Design review of the part built by this model. Coordinates are the model's own, in mm. A direction names the side the tool comes from. Coordinates: 2 decimals unless noted, no trailing zeros. Order: outer loops, then holes, each group sorted by start corner. A loop starts at its lowest first (then second) coordinate and runs counter-clockwise, first axis right, second up. Notation, with made-up numbers: M 83,72 L 127,72 A5 cw 127,78 Z; hole C 15.25,58.5 d4. An arc over 180 degrees is marked long. Answer as a JSON object with one key per item and string values.
from build123d import *

# Parameters (mm, degrees)
MODEL_R             = 19.83955
BOSS_EXTRUDE1_DEPTH = 6.35


with BuildPart() as part:
    # Model → Boss-Extrude1 (new body)
    with BuildSketch(Plane.XY):
        with BuildLine():
            Line((-20.5954, 56.0124), (-20.5954, 81.2129))
            Line((-20.5954, 81.2129), (-14.4452, 81.2129))
            Line((-14.4452, 81.2129), (-14.4452, 107.2136))
            Line((-14.4452, 107.2136), (-20.5954, 107.2136))
            Line((-20.5954, 107.2136), (-20.5954, 132.4124))
            Line((-20.5954, 132.4124), (-14.4452, 132.4124))
            Line((-14.4452, 132.4124), (-14.4452, 151.262))
            Line((-14.4452, 151.262), (-4.2849, 151.262))
            Line((-4.2849, 151.262), (-4.2849, 161.223))
            add(Edge.make_bspline(
                [(2.0647, 167.573), (-1.4529, 167.573), (-4.2849, 164.741), (-4.2849, 161.223)],
                knots=[0.181818182, 0.181818182, 0.181818182, 0.181818182, 0.212121212, 0.212121212, 0.212121212, 0.212121212], degree=3))
            Line((2.0647, 167.573), (27.2651, 167.573))
            add(Edge.make_bspline(
                [(33.6151, 161.223), (33.6151, 164.741), (30.7835, 167.573), (27.2651, 167.573)],
                knots=[0.121212121, 0.121212121, 0.121212121, 0.121212121, 0.151515152, 0.151515152, 0.151515152, 0.151515152], degree=3))
            Line((33.6151, 161.223), (33.6151, 151.262))
            Line((33.6151, 151.262), (43.7754, 151.262))
            Line((43.7754, 151.262), (43.7754, 132.4124))
            Line((43.7754, 132.4124), (49.9256, 132.4124))
            Line((49.9256, 132.4124), (49.9256, 107.2136))
            Line((49.9256, 107.2136), (43.7754, 107.2136))
            Line((43.7754, 107.2136), (43.7754, 81.2129))
            Line((43.7754, 81.2129), (49.9256, 81.2129))
            Line((49.9256, 81.2129), (49.9256, 56.0124))
            Line((49.9256, 56.0124), (43.7754, 56.0124))
            Line((43.7754, 56.0124), (43.7754, 37.1628))
            Line((43.7754, 37.1628), (33.6151, 37.1628))
            Line((33.6151, 37.1628), (33.6151, 27.2034))
            add(Edge.make_bspline(
                [(27.2651, 20.8535), (30.7835, 20.8535), (33.6151, 23.6854), (33.6151, 27.2034)],
                knots=[0.666666667, 0.666666667, 0.666666667, 0.666666667, 0.696969697, 0.696969697, 0.696969697, 0.696969697], degree=3))
            Line((27.2651, 20.8535), (2.0647, 20.8535))
            add(Edge.make_bspline(
                [(-4.2849, 27.2034), (-4.2849, 23.6854), (-1.4529, 20.8535), (2.0647, 20.8535)],
                knots=[0.606060606, 0.606060606, 0.606060606, 0.606060606, 0.636363636, 0.636363636, 0.636363636, 0.636363636], degree=3))
            Line((-4.2849, 27.2034), (-4.2849, 37.1628))
            Line((-4.2849, 37.1628), (-14.4452, 37.1628))
            Line((-14.4452, 37.1628), (-14.4452, 56.0124))
            Line((-14.4452, 56.0124), (-20.5954, 56.0124))
        make_face()
        with Locations((14.6645, 94.21325)):
            Circle(MODEL_R, mode=Mode.SUBTRACT)
        with BuildLine():
            Line((-6.1122, 70.2543), (-8.1775, 68.1903))
            add(Edge.make_bspline(
                [(-8.1775, 68.1903), (-9.0583, 67.3086), (-10.4778, 67.3086), (-11.3583, 68.1903)],
                knots=[0.142857143, 0.142857143, 0.142857143, 0.142857143, 0.285714286, 0.285714286, 0.285714286, 0.285714286], degree=3))
            add(Edge.make_bspline(
                [(-11.3583, 68.1903), (-12.2399, 69.0707), (-12.2399, 70.4906), (-11.3583, 71.3711)],
                knots=[0.285714286, 0.285714286, 0.285714286, 0.285714286, 0.428571429, 0.428571429, 0.428571429, 0.428571429], degree=3))
            Line((-11.3583, 71.3711), (-9.293, 73.4364))
            add(Edge.make_bspline(
                [(-9.293, 73.4364), (-8.4121, 74.3185), (-6.9926, 74.3185), (-6.1122, 73.4364)],
                knots=[0.571428571, 0.571428571, 0.571428571, 0.571428571, 0.714285714, 0.714285714, 0.714285714, 0.714285714], degree=3))
            add(Edge.make_bspline(
                [(-6.1122, 73.4364), (-5.2301, 72.5559), (-5.2301, 71.1364), (-6.1122, 70.2543)],
                knots=[0.714285714, 0.714285714, 0.714285714, 0.714285714, 1, 1, 1, 1], degree=3))
        make_face(mode=Mode.SUBTRACT)
        with BuildLine():
            Line((40.6885, 117.0554), (38.6232, 114.9897))
            add(Edge.make_bspline(
                [(38.6232, 114.9897), (37.7415, 114.1092), (36.3232, 114.1092), (35.4411, 114.9897)],
                knots=[0.142857143, 0.142857143, 0.142857143, 0.142857143, 0.285714286, 0.285714286, 0.285714286, 0.285714286], degree=3))
            add(Edge.make_bspline(
                [(35.4411, 114.9897), (34.5607, 115.8705), (34.5607, 117.29), (35.4411, 118.1717)],
                knots=[0.285714286, 0.285714286, 0.285714286, 0.285714286, 0.428571429, 0.428571429, 0.428571429, 0.428571429], degree=3))
            Line((35.4411, 118.1717), (37.5068, 120.2357))
            add(Edge.make_bspline(
                [(37.5068, 120.2357), (38.3885, 121.1178), (39.8068, 121.1178), (40.6889, 120.2357)],
                knots=[0.571428571, 0.571428571, 0.571428571, 0.571428571, 0.714285714, 0.714285714, 0.714285714, 0.714285714], degree=3))
            add(Edge.make_bspline(
                [(40.6889, 120.2357), (41.5693, 119.3553), (41.5693, 117.9358), (40.6885, 117.0554)],
                knots=[0.714285714, 0.714285714, 0.714285714, 0.714285714, 1, 1, 1, 1], degree=3))
        make_face(mode=Mode.SUBTRACT)
        with BuildLine():
            Line((40.6885, 71.3707), (38.6227, 73.4364))
            add(Edge.make_bspline(
                [(38.6227, 73.4364), (37.7411, 74.3185), (36.3228, 74.3185), (35.4407, 73.4364)],
                knots=[0.142857143, 0.142857143, 0.142857143, 0.142857143, 0.285714286, 0.285714286, 0.285714286, 0.285714286], degree=3))
            add(Edge.make_bspline(
                [(35.4407, 73.4364), (34.5603, 72.5559), (34.5607, 71.1368), (35.4411, 70.2547)],
                knots=[0.285714286, 0.285714286, 0.285714286, 0.285714286, 0.428571429, 0.428571429, 0.428571429, 0.428571429], degree=3))
            Line((35.4411, 70.2547), (37.5068, 68.1903))
            add(Edge.make_bspline(
                [(37.5068, 68.1903), (38.3889, 67.3086), (39.8064, 67.3086), (40.6885, 68.1903)],
                knots=[0.571428571, 0.571428571, 0.571428571, 0.571428571, 0.714285714, 0.714285714, 0.714285714, 0.714285714], degree=3))
            add(Edge.make_bspline(
                [(40.6885, 68.1903), (41.5689, 69.0707), (41.5693, 70.4902), (40.6885, 71.3707)],
                knots=[0.714285714, 0.714285714, 0.714285714, 0.714285714, 1, 1, 1, 1], degree=3))
        make_face(mode=Mode.SUBTRACT)
        with BuildLine():
            Line((-6.1122, 118.1717), (-8.1766, 120.2357))
            add(Edge.make_bspline(
                [(-8.1766, 120.2357), (-9.0587, 121.1178), (-10.4782, 121.1178), (-11.3587, 120.2357)],
                knots=[0.142857143, 0.142857143, 0.142857143, 0.142857143, 0.285714286, 0.285714286, 0.285714286, 0.285714286], degree=3))
            add(Edge.make_bspline(
                [(-11.3587, 120.2357), (-12.2391, 119.3553), (-12.2387, 117.9362), (-11.3583, 117.0554)],
                knots=[0.285714286, 0.285714286, 0.285714286, 0.285714286, 0.428571429, 0.428571429, 0.428571429, 0.428571429], degree=3))
            Line((-11.3583, 117.0554), (-9.2926, 114.9897))
            add(Edge.make_bspline(
                [(-9.2926, 114.9897), (-8.4121, 114.1076), (-6.993, 114.1076), (-6.1126, 114.9897)],
                knots=[0.571428571, 0.571428571, 0.571428571, 0.571428571, 0.714285714, 0.714285714, 0.714285714, 0.714285714], degree=3))
            add(Edge.make_bspline(
                [(-6.1126, 114.9897), (-5.2305, 115.8705), (-5.2301, 117.2896), (-6.1122, 118.1717)],
                knots=[0.714285714, 0.714285714, 0.714285714, 0.714285714, 1, 1, 1, 1], degree=3))
        make_face(mode=Mode.SUBTRACT)
        with BuildLine():
            add(Edge.make_bspline(
                [(8.6945, 154.6937), (10.0978, 154.6937), (11.2349, 155.8307), (11.2349, 157.2336)],
                knots=[0, 0, 0, 0, 0.2, 0.2, 0.2, 0.2], degree=3))
            add(Edge.make_bspline(
                [(11.2349, 157.2336), (11.2349, 158.6365), (10.0978, 159.7728), (8.6945, 159.7728)],
                knots=[0.2, 0.2, 0.2, 0.2, 0.4, 0.4, 0.4, 0.4], degree=3))
            add(Edge.make_bspline(
                [(8.6945, 159.7728), (7.2921, 159.7728), (6.1537, 158.6365), (6.1537, 157.2336)],
                knots=[0.4, 0.4, 0.4, 0.4, 0.6, 0.6, 0.6, 0.6], degree=3))
            add(Edge.make_bspline(
                [(6.1537, 157.2336), (6.1537, 155.8307), (7.2921, 154.6937), (8.6945, 154.6937)],
                knots=[0.6, 0.6, 0.6, 0.6, 1, 1, 1, 1], degree=3))
        make_face(mode=Mode.SUBTRACT)
        with BuildLine():
            add(Edge.make_bspline(
                [(8.6945, 28.6532), (10.0978, 28.6532), (11.2349, 29.7899), (11.2349, 31.1928)],
                knots=[0, 0, 0, 0, 0.2, 0.2, 0.2, 0.2], degree=3))
            add(Edge.make_bspline(
                [(11.2349, 31.1928), (11.2349, 32.5953), (10.0978, 33.7324), (8.6945, 33.7324)],
                knots=[0.2, 0.2, 0.2, 0.2, 0.4, 0.4, 0.4, 0.4], degree=3))
            add(Edge.make_bspline(
                [(8.6945, 33.7324), (7.2921, 33.7324), (6.1537, 32.5953), (6.1537, 31.1928)],
                knots=[0.4, 0.4, 0.4, 0.4, 0.6, 0.6, 0.6, 0.6], degree=3))
            add(Edge.make_bspline(
                [(6.1537, 31.1928), (6.1537, 29.7899), (7.2921, 28.6532), (8.6945, 28.6532)],
                knots=[0.6, 0.6, 0.6, 0.6, 1, 1, 1, 1], degree=3))
        make_face(mode=Mode.SUBTRACT)
        with BuildLine():
            add(Edge.make_bspline(
                [(20.6352, 154.6937), (22.0385, 154.6937), (23.1752, 155.8307), (23.1752, 157.2336)],
                knots=[0, 0, 0, 0, 0.2, 0.2, 0.2, 0.2], degree=3))
            add(Edge.make_bspline(
                [(23.1752, 157.2336), (23.1752, 158.6365), (22.0385, 159.7728), (20.6352, 159.7728)],
                knots=[0.2, 0.2, 0.2, 0.2, 0.4, 0.4, 0.4, 0.4], degree=3))
            add(Edge.make_bspline(
                [(20.6352, 159.7728), (19.2328, 159.7728), (18.0957, 158.6365), (18.0957, 157.2336)],
                knots=[0.4, 0.4, 0.4, 0.4, 0.6, 0.6, 0.6, 0.6], degree=3))
            add(Edge.make_bspline(
                [(18.0957, 157.2336), (18.0957, 155.8307), (19.2328, 154.6937), (20.6352, 154.6937)],
                knots=[0.6, 0.6, 0.6, 0.6, 1, 1, 1, 1], degree=3))
        make_face(mode=Mode.SUBTRACT)
        with BuildLine():
            add(Edge.make_bspline(
                [(20.6352, 28.6532), (22.0385, 28.6532), (23.1752, 29.7899), (23.1752, 31.1928)],
                knots=[0, 0, 0, 0, 0.2, 0.2, 0.2, 0.2], degree=3))
            add(Edge.make_bspline(
                [(23.1752, 31.1928), (23.1752, 32.5953), (22.0385, 33.7324), (20.6352, 33.7324)],
                knots=[0.2, 0.2, 0.2, 0.2, 0.4, 0.4, 0.4, 0.4], degree=3))
            add(Edge.make_bspline(
                [(20.6352, 33.7324), (19.2328, 33.7324), (18.0957, 32.5953), (18.0957, 31.1928)],
                knots=[0.4, 0.4, 0.4, 0.4, 0.6, 0.6, 0.6, 0.6], degree=3))
            add(Edge.make_bspline(
                [(18.0957, 31.1928), (18.0957, 29.7899), (19.2328, 28.6532), (20.6352, 28.6532)],
                knots=[0.6, 0.6, 0.6, 0.6, 1, 1, 1, 1], degree=3))
        make_face(mode=Mode.SUBTRACT)
        with BuildLine():
            add(Edge.make_bspline(
                [(14.6645, 129.7262), (16.0674, 129.7262), (17.2053, 130.8633), (17.2053, 132.2662)],
                knots=[0, 0, 0, 0, 0.2, 0.2, 0.2, 0.2], degree=3))
            add(Edge.make_bspline(
                [(17.2053, 132.2662), (17.2053, 133.6691), (16.0674, 134.8074), (14.6645, 134.8074)],
                knots=[0.2, 0.2, 0.2, 0.2, 0.4, 0.4, 0.4, 0.4], degree=3))
            add(Edge.make_bspline(
                [(14.6645, 134.8074), (13.2616, 134.8074), (12.1245, 133.6691), (12.1245, 132.2662)],
                knots=[0.4, 0.4, 0.4, 0.4, 0.6, 0.6, 0.6, 0.6], degree=3))
            add(Edge.make_bspline(
                [(12.1245, 132.2662), (12.1245, 130.8633), (13.2616, 129.7262), (14.6645, 129.7262)],
                knots=[0.6, 0.6, 0.6, 0.6, 1, 1, 1, 1], degree=3))
        make_face(mode=Mode.SUBTRACT)
        with BuildLine():
            add(Edge.make_bspline(
                [(14.6645, 53.5264), (16.0674, 53.5264), (17.2053, 54.6635), (17.2053, 56.0664)],
                knots=[0, 0, 0, 0, 0.2, 0.2, 0.2, 0.2], degree=3))
            add(Edge.make_bspline(
                [(17.2053, 56.0664), (17.2053, 57.4693), (16.0674, 58.6076), (14.6645, 58.6076)],
                knots=[0.2, 0.2, 0.2, 0.2, 0.4, 0.4, 0.4, 0.4], degree=3))
            add(Edge.make_bspline(
                [(14.6645, 58.6076), (13.2616, 58.6076), (12.1245, 57.4693), (12.1245, 56.0664)],
                knots=[0.4, 0.4, 0.4, 0.4, 0.6, 0.6, 0.6, 0.6], degree=3))
            add(Edge.make_bspline(
                [(12.1245, 56.0664), (12.1245, 54.6635), (13.2616, 53.5264), (14.6645, 53.5264)],
                knots=[0.6, 0.6, 0.6, 0.6, 1, 1, 1, 1], degree=3))
        make_face(mode=Mode.SUBTRACT)
    extrude(amount=BOSS_EXTRUDE1_DEPTH)


solid = part.part
1) Add section B-B (y = 83). State the section outline as (x, z) points.
Taken from the geometry:
{"outline": "M -14.45,0 L -1.7,0 L -1.7,6.35 L -14.45,6.35 Z; M 31.03,0 L 43.78,0 L 43.78,6.35 L 31.03,6.35 Z"}
2) Insertion check: pin 1 Ø1.9 at (x, z) = (-10, 3.5) entering from -Y; pin 2 Ø1.5 at (x, y) = (-9.5, 72.5) entering from +Z; pin 3 Ø1.9 at (y, z) = (141, 1.5) entering from -X; pin 4 Ø3 at (y, z) = (98.5, 5.5) entering from +X. Each pin has a flat end and moves straight along its axis. Give the tip position at first contact, or say it passes through.
Taken from the geometry:
{"pin 1": "stops at y = 37.16", "pin 2": "stops at z = 6.35", "pin 3": "stops at x = -14.45", "pin 4": "stops at x = 43.78"}
3) Add section C-C (y = 138). State the section outline as (x, z) points, and give its area (3 significant figures).
Taken from the geometry:
{"outline": "M -14.45,0 L 43.78,0 L 43.78,6.35 L -14.45,6.35 Z", "area": "370 mm2"}
4) Add section D-D (x = 21.5). Count the separate pieces of the cut face and the enclosed holes in it, and give its area (3 significant figures).
Taken from the geometry:
{"separate pieces": "4", "enclosed holes": "0", "area": "634 mm2"}
5) Mouldability with a two-part tool opening along Y and no side actions: class faces 1 (the flat face through (47, 107.214, 3)), 2 (the flat face through (14, 167.573, 3)), 3 (the flat face through (-4.285, 156, 3)), 4 (the flat face through (47, 56.012, 3)) as released by +Y, released by -Y, zero draft, split by the parting line, or undercut.
Taken from the geometry:
{"face 1": "undercut", "face 2": "released by +Y", "face 3": "zero draft", "face 4": "released by -Y"}
6) To check wall thickness, follow L1, parallel to Y at x = -17, z = 5.5; L2, parallel to Y at x = 10, z = 3.5; L3, parallel to Y at x = -9, z = 5. State the ranges of each line that lie inside material, in increasing order.
Taken from the geometry:
{"L1": "y = 56.01 to 81.21, 107.21 to 132.41", "L2": "y = 20.85 to 29.01, 33.37 to 74.93, 113.5 to 155.05, 159.41 to 167.57", "L3": "y = 37.16 to 67.66, 73.68 to 114.74, 120.76 to 151.26"}
7) Tool access review of faces 5 (the flat face through (-9, 151.262, 3)), 6 (the flat face through (33.615, 156, 3)), 7 (the flat face through (-17, 56.012, 3)): name each direction out of +Z, -Z, +X, -X, +Y, -Y from which nothing blocks a thin tool from reaching the whole face with its end or side.
Taken from the geometry:
{"face 5": "+Z, -Z, -X, +Y", "face 6": "+Z, -Z, +X, +Y", "face 7": "+Z, -Z, -X, -Y"}
8) Add section A-A (x = 46.5). State the section outline as (y, z) points.
Taken from the geometry:
{"outline": "M 56.01,0 L 81.21,0 L 81.21,6.35 L 56.01,6.35 Z; M 107.21,0 L 132.41,0 L 132.41,6.35 L 107.21,6.35 Z"}
